from build123d import *

# Parameters (mm, degrees)
SKETCH1_W           = 50.8
SKETCH1_H           = 50.8
BOSS_EXTRUDE1_DEPTH = 38.1
SKETCH3_R           = 5.588
CUT_EXTRUDE1_DEPTH  = 25.4
SKETCH4_R           = 4.7625
CUT_EXTRUDE2_DEPTH  = 51.8


with BuildPart() as part:
    # Sketch1 → Boss-Extrude1 (new body)
    with BuildSketch(Plane.XY):
        Rectangle(SKETCH1_W, SKETCH1_H)
    extrude(amount=BOSS_EXTRUDE1_DEPTH)

    # Sketch3 → Cut-Extrude1 (cut)
    with BuildSketch(Plane.XZ.offset(25.4)):
        with Locations((0, 19.05)):
            Circle(SKETCH3_R)
    extrude(amount=-CUT_EXTRUDE1_DEPTH, mode=Mode.SUBTRACT)

    # Sketch4 → Cut-Extrude2 (cut, through all)
    with BuildSketch(Plane.ZY.offset(25.4)):
        with Locations((18.915028582, 12.7)):
            Circle(SKETCH4_R)
    extrude(amount=-CUT_EXTRUDE2_DEPTH, mode=Mode.SUBTRACT)


solid = part.part
Design review of the part built by this model. Coordinates are the model's own, in mm. A direction names the side the tool comes from. Coordinates: 2 decimals unless noted, no trailing zeros. Loops run counter-clockwise (first coordinate to the right, second up) from the corner with the lowest first, then second, coordinate; pieces in that order, holes last. Notation, with made-up numbers: (47, 5.25) -> (58, 5.25) arc R6 ccw to (58, 14.25) -> close; hole circle Ø10 at (86, 20). An arc over 180 degrees is marked (long way). Use a Markdown table: item, result. Add a question column.
Item 1: Machinability: for faces 5 (the flat face through (0, 0, 38.1)), 6 (the flat face through (0, 0, 19)), which of the approach directions +Z, -Z, +X, -X, +Y, -Y give a long, thin tool a straight path to every point of the face, cutting with its end or side? Answer none if there is none.
Item 2: Wall thickness on L1, parallel to Z at x = 0, y = -8.5; L2, parallel to X at y = -5, z = 19; L3, parallel to Y at x = 13, z = 16: over which ranges is each line inside the solid? List them lowest first. Write a range as from..to.
Item 3: Clearance check with a flat-ended pin moving along its axis: P1, Ø3.5, axis at x = 2, z = 18.5, coming from the -Y side. State where the tip first meets the part, or that it passes through.
Item 4: The part is to be moulded in two halves that separate along Z. For faces 1 (the flat face through (0, 0, 0)), 2 (the cylindrical face through (-0.356, 12.909, 14.157)), 3 (the cylindrical face through (-1.211, -12.878, 13.595)), 4 (the flat face through (25.4, 0, 19)), say which applies: +Z half, -Z half, draft (parallel to the pull), parting line (faces both ways), or undercut.
Item 5: We need section B-B, the plane y = 12. Write out the cut boundary in (x, z).
Item 6: We need section C-C, the plane z = 19.05. Write out the cut boundary in (x, y), and give its area (3 significant figures).
Item 7: We need section D-D, the plane y = -1. Write out the cut boundary in (x, z), and give its area (3 significant figures).
Numbers:
| question | item | result |
|---|---|---|
| 1 | face 5 | +Z, +X, -X, +Y, -Y |
| 1 | face 6 | -Y |
| 2 | L1 | z = 0..13.46, 24.64..38.1 |
| 2 | L2 | x = -25.4..-5.59, 5.59..25.4 |
| 2 | L3 | y = -25.4..8.93, 16.47..25.4 |
| 3 | P1 | stops at y = 0 |
| 4 | face 1 | -Z half |
| 4 | face 2 | undercut |
| 4 | face 3 | undercut |
| 4 | face 4 | draft |
| 5 | outline | (-25.4, 0) -> (25.4, 0) -> (25.4, 14.2) -> (-25.4, 14.2) -> close; (-25.4, 23.63) -> (25.4, 23.63) -> (25.4, 38.1) -> (-25.4, 38.1) -> close |
| 6 | outline | (-25.4, -25.4) -> (-5.59, -25.4) -> (-5.59, 0) -> (5.59, 0) -> (5.59, -25.4) -> (25.4, -25.4) -> (25.4, 7.94) -> (-25.4, 7.94) -> close; (-25.4, 17.46) -> (25.4, 17.46) -> (25.4, 25.4) -> (-25.4, 25.4) -> close |
| 6 | area | 1,810 mm^2 |
| 7 | outline | (-25.4, 0) -> (25.4, 0) -> (25.4, 38.1) -> (-25.4, 38.1) -> close; hole circle Ø11.18 at (0, 19.05) |
| 7 | area | 1,840 mm^2 |
